Autodesk Inventor part; units mm, degrees
ref_plane "YZ Plane" through (0, 0, 0) normal (1, 0, 0) x (0, 1, 0)
ref_plane "XZ Plane" through (0, 0, 0) normal (0, 1, 0) x (-1, 0, 0)
ref_plane "XY Plane" through (0, 0, 0) normal (0, 0, 1) x (1, 0, 0)
sketch "Sketch1" plane through (0, 0, 0) normal (0, 0, 1) x (1, 0, 0)
  circle A0 centre (0, 0) radius 12.5
  line L0 (12.5, 0) -> (12.5, 22.5)
  line L1 (12.5, 22.5) -> (-22.5, 22.5)
  line L2 (-22.5, 22.5) -> (-22.5, -12.5)
  line L3 (-22.5, -12.5) -> (0, -12.5)
  dimension "d0" = 25
  dimension "d1" = 35
  dimension "d2" = 35
extrude "Extrusion1" add sketch "Sketch1" along normal blind 25
draft "FaceDraft1" angle 2.5 pull direction (0, 0, 1) faces at (-15, -12.5, 8.3333) (3.6844, -11.9447, 16.6667) (12.5, 7.5, 8.3333) fixed edges at (-11.25, -12.5, 0) (8.8388, -8.8388, 0) (12.5, 11.25, 0)
sketch "Sketch2" plane through (0, 0, 0) normal (0, 0, -1) x (-1, 0, 0)
  circle A0 centre (0, 0) radius 2.75
  dimension "d6" = 5.5
extrude "Extrusion2" cut sketch "Sketch2" against normal through all
ref_plane "Work Plane1" through (0, 0, 10) normal (0, 0, -1) x (-1, 0, 0)
sketch "Sketch3" plane through (0, 0, 25) normal (0, 0, 1) x (1, 0, 0)
  circle A0 centre (0, 0) radius 2.75
  circle A1 centre (0, 0) radius 7.5
  dimension "d10" = 15
extrude "Extrusion3" cut sketch "Sketch3" against normal up to surface (15 mm away)
chamfer "Chamfer1" distance 1 angle 45 6 edges at (8.8388, -8.8388, 0) (12.5, 11.25, 0) (-11.25, -12.5, 0) (2.75, 0, 0) (-5, 22.5, 0) (-22.5, 5, 0)
sketch "Sketch4" plane through (0, 0, 25) normal (0, 0, 1) x (1, 0, 0)
  line L0 (12.4564, 22.499) -> (12.4564, 0)
  line L1 (0, -12.4564) -> (-22.499, -12.4564)
  line L2 (12.4564, 9.5436) -> (-9.5436, 9.5436)
  line L3 (-9.5436, -12.4564) -> (-9.5436, 9.5436)
  arc A0 (0, -12.4564) -> (12.4564, 0) centre (0, 0) ccw
  line L4 (22, -23) -> (-37, -23)
  line L5 (-37, -23) -> (-37, 27)
  line L6 (-37, 27) -> (22, 27)
  line L7 (22, 27) -> (22, -23)
  point P0 (0, 0)
  dimension "d16" = 22
  dimension "d17" = 22
extrude "Extrusion4" cut sketch "Sketch4" against normal through all
fillet "Fillet1" radius 2 2 edges at (-9.5436, -11.9324, 12.9995) (11.9324, 9.5436, 12.9995)
equation "\"d2\" = d1"
equation "\"d17\" = d16"
properties part number "CornerHolder_3DPrint"
Part model, mm, in its own coordinate system. A direction names the side the tool comes from. Give positions to 0.01 mm unless a question says otherwise; leave off trailing zeros. Loops run counter-clockwise (first coordinate to the right, second up) from the corner with the lowest first, then second, coordinate; pieces in that order, holes last. Notation, with made-up numbers: M -20,-20.5 L 12,-20.5 A19 cw 12,4.5 Z; hole C 20,-14.5 d4. An arc over 180 degrees is marked long. Put each result on its own line as item: value. Start each with the question number.
1) Saw through at A-A (y = 6.25). List the corners of the cut face in (x, z).
2) Probe probe 1 along X at (y, z) = (0, 7); probe 2 along Z at (x, y) = (-6.75, -2.25); probe 3 along Y at (x, z) = (0, 15.5). List the from-to ranges inside material, lowest first.
3) Pull direction X, two halves, no side cores. Call faces 1 (the cylindrical face through (-8.94, -11.39, 12.37)), 2 (the flat face through (5.44, -5.44, 25)), 3 (the cylindrical face through (0.596, -2.685, 5.437)): +X half, -X half, draft (parallel to the pull), parting line (faces both ways), or undercut.
4) 3-axis set-ups, long thin cutter, end or side, ignore diameter. For faces 4 (the conical face through (8.158, -8.339, 0.174)), 5 (the flat face through (0, -3, 10)): which of +Z, -Z, +X, -X, +Y, -Y reach the whole face in a straight line?
5) Flat gauge pins, fed straight in: pin 1 (1 mm diameter, centred on x = -3, y = 0.5, fed in from +Z); pin 2 (1.5 mm diameter, centred on y = 6, z = 16, fed in from +X); pin 3 (1 mm diameter, centred on x = -2, y = 2, fed in from -Z). Where does each tip first touch, or does it go through?
Numbers:
1. outline: M -9.54,0 L 11.5,0 L 12.46,1 L 11.41,25 L 4.15,25 L 4.15,10 L -4.15,10 L -4.15,25 L -9.54,25 Z
2. probe 1: -9.54 to -2.75, 2.75 to 12.19
2. probe 2: 0 to 10
2. probe 3: -11.82 to -7.5, 7.5 to 9.54
3. face 1: -X half
3. face 2: draft
3. face 3: undercut
4. face 4: -Z, +X, -Y
4. face 5: +Z
5. pin 1: z = 10
5. pin 2: x = 11.83
5. pin 3: z = 0.42
